Verification items for the finished model (mm, model axes). Face numbers are marked on the shaded views. Give positions to 0.01 mm unless a question says otherwise; leave off trailing zeros. Write each loop counter-clockwise with the first axis right and the second up, starting at its lowest first coordinate (ties: lowest second). Pieces come first, ordered by that corner, then holes. Notation, with made-up numbers: (-38.75, -32.5) -> (-12.75, -32.5) arc R28 cw to (-12.75, 5.5) -> close; hole circle Ø5 at (45, 20.5). An arc over 180 degrees is marked (long way). Answer as CSV lines item,"result". Start each with the question number.
1) Gauge pin test, flat ends, axial feed: pin 1 Ø1 at (x, y) = (22, -1.5) entering from +Z; pin 2 Ø5 at (x, z) = (1, 2.5) entering from +Y; pin 3 Ø2 at (x, z) = (28, 8) entering from +Y. Record the tip position at first contact, or that the pin passes through.
2) Sectioned sample at B-B on x = -29.5. Record the cut outline in (y, z) (3 decimals), and give its area (3 significant figures).
3) Material ranges on L1, parallel to X at y = 7, z = -19.5; L2, parallel to X at y = -25.5, z = 11; L3, parallel to Y at x = 31.5, z = -6, recorded low to high.
4) Sectioned sample at A-A on z = 0. Record the cut outline in (x, y), and give its area (3 significant figures).
5) Mould release check, pull along X, two halves, no side actions. Record for the marked faces 1, 2 and 3: released by +X, released by -X, zero draft, split by the parting line, or undercut.
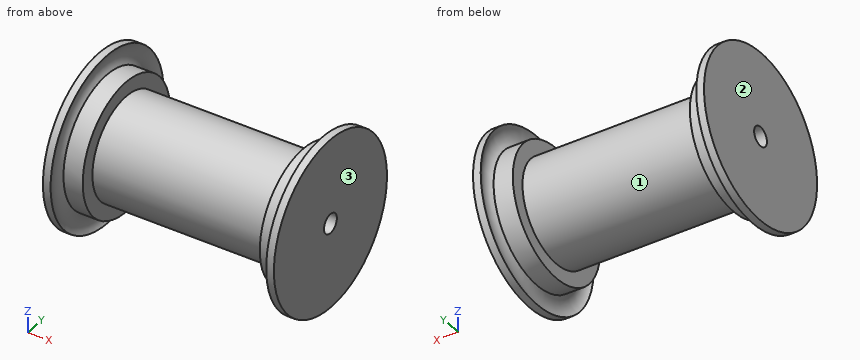
Autodesk Inventor part; units mm, degrees
ref_plane "YZ Plane" through (0, 0, 0) normal (1, 0, 0) x (0, 1, 0)
ref_plane "XZ Plane" through (0, 0, 0) normal (0, 1, 0) x (-1, 0, 0)
ref_plane "XY Plane" through (0, 0, 0) normal (0, 0, 1) x (1, 0, 0)
sketch "Sketch1" plane through (0, 0, 0) normal (0, 0, 1) x (1, 0, 0)
  line L0 (-36.4853, -0.2751) -> (39.7147, -0.2751)
  line L1 (-36.4853, -0.2751) -> (-36.4853, 27.6649)
  line L2 (-36.4853, 27.6649) -> (-33.9453, 27.6649)
  arc A0 (-33.9453, 27.6649) -> (-33.9453, 21.3149) centre (-29.9798, 24.4899) ccw
  line L3 (-33.9453, 21.3149) -> (-27.5953, 21.3149)
  line L4 (-27.5953, 21.3149) -> (-27.5953, 16.5345)
  line L5 (39.7147, -0.2751) -> (39.7147, 27.6649)
  line L6 (39.7147, 27.6649) -> (37.1747, 27.6649)
  arc A1 (37.1747, 21.3149) -> (37.1747, 27.6649) centre (33.2091, 24.4899) ccw
  line L7 (37.1747, 21.3149) -> (30.8247, 21.3149)
  line L8 (30.8247, 21.3149) -> (30.8247, 16.5345)
  line L9 (-27.5953, 16.5345) -> (30.8247, 16.5345)
  point P0 (0, 0)
  dimension "d0" = 76.2
  dimension "d1" = 27.94
  dimension "d2" = 2.54
  dimension "d3" = 6.35
  dimension "d4" = 5.08
  dimension "d5" = 6.35
revolve "Revolution1" add sketch "Sketch1" angle 360 about axis through (-36.4853, -0.2751, 0) along (1, 0, 0)
sketch "Sketch2" plane through (0, 0, 0) normal (1, 0, 0) x (0, 1, 0)
  circle A0 centre (0, 0) radius 3.175
  circle A1 centre (0, 0) radius 3.175
sketch "Sketch3" plane through (-36.4853, -0.2751, 0) normal (-1, 0, 0) x (0, 0, 1)
  circle A0 centre (0, 0.2751) radius 3.175
  circle A1 centre (0, 0) radius 27.94
  dimension "d9" = 6.35
  dimension "d10" = 25.0401
hole "Hole1" at (-36.4853, -0.2751, 0) direction (1, 0, 0) diameter 6.35 end through all both
sketch "Sketch4" plane through (-36.4853, -0.2751, 0) normal (-1, 0, 0) x (0, 0, 1)
  point P0 (0, 0.2751)
sketch "Sketch5" plane through (-36.4853, -0.2751, 0) normal (-1, 0, 0) x (0, 0, 1)
  point P0 (0, 0.2751)
sketch "Sketch6" plane through (39.7147, -0.2751, 0) normal (1, 0, 0) x (0, 0, -1)
  point P0 (0, 0.2751)
sketch "Sketch7" plane through (0, 0, 0) normal (1, 0, 0) x (0, 1, 0)
  point P0 (0, 0)
properties part number "weel 2.2"
Ans:
1,pin 1,"stops at z = 16.79"
1,pin 2,"stops at y = 16.53"
1,pin 3,"stops at y = 15.01"
2,outline,"circle Ø43.18 at (-0.275, 0); hole circle Ø6.35 at (-0.275, 0)"
2,area,"1,430 mm²"
3,L1,"x = -36.49 to -27.6, 30.82 to 39.71"
3,L2,"x = -36.49 to -34.25, 37.48 to 39.71"
3,L3,"y = -21.01 to 20.46"
4,outline,"(-36.49, -28.22) -> (-33.95, -28.22) arc R5.08 cw to (-33.95, -21.87) -> (-27.6, -21.87) -> (-27.6, -17.08) -> (30.82, -17.08) -> (30.82, -21.87) -> (37.17, -21.87) arc R5.08 cw to (37.17, -28.22) -> (39.71, -28.22) -> (39.71, -3.45) -> (-36.49, -3.45) -> close; (-36.49, 2.9) -> (39.71, 2.9) -> (39.71, 27.66) -> (37.17, 27.66) arc R5.08 cw to (37.17, 21.31) -> (30.82, 21.31) -> (30.82, 16.53) -> (-27.6, 16.53) -> (-27.6, 21.31) -> (-33.95, 21.31) arc R5.08 cw to (-33.95, 27.66) -> (-36.49, 27.66) -> close"
4,area,"2,290 mm²"
5,face 1,"undercut"
5,face 2,"released by -X"
5,face 3,"released by +X"
